Geometry check sheet. Reference: the model listing, model coordinates, mm. A direction names the side the tool comes from. Round coordinates to 2 decimals unless told otherwise and drop trailing zeros. Loops run counter-clockwise (first coordinate to the right, second up) from the corner with the lowest first, then second, coordinate; pieces in that order, holes last.
```python
from build123d import *

# Parameters (mm, degrees)
F1_DEPTH = 25.4
F2_DEPTH = 25.4
F3_DEPTH = 25.4


with BuildPart() as f1:
    # F0 (on Front) → F1 (new body)
    with BuildSketch(Plane.XZ):
        with BuildLine():
            ThreePointArc((-119.86399662, 0), (-111.5302178098, 16.6558061897), (-108.6615478184, 35.0579387173))
            ThreePointArc((-108.6615478184, 35.0579387173), (-111.4781642304, 53.2963683876), (-119.6655722325, 69.8354129505))
            Line((-119.6655722325, 69.8354129505), (-201.6532506958, 69.8354129505))
            Line((-201.6532506958, 69.8354129505), (-201.6532506958, 0))
            Line((-201.6532506958, 0), (-119.86399662, 0))
        make_face()
        with BuildLine():
            ThreePointArc((-119.6655722325, 69.8354129505), (-111.4781642304, 53.2963683876), (-108.6615478184, 35.0579387173))
            ThreePointArc((-108.6615478184, 35.0579387173), (-111.5302178098, 16.6558061897), (-119.86399662, 0))
            Line((-119.86399662, 0), (86.1022950306, 0))
            Line((86.1022950306, 0), (86.1022950306, 69.8354129505))
            Line((86.1022950306, 69.8354129505), (-119.6655722325, 69.8354129505))
        make_face()
        with BuildLine():
            Line((-201.6532506958, 69.8354129505), (-119.6655722325, 69.8354129505))
            ThreePointArc((-119.6655722325, 69.8354129505), (-229.5771812139, 35.2297180557), (-119.86399662, 0))
            Line((-119.86399662, 0), (-201.6532506958, 0))
            Line((-201.6532506958, 0), (-201.6532506958, 69.8354129505))
        make_face()
    extrude(amount=F1_DEPTH)

    # F2 (add): a face of the model
    f2_faces = [f1.faces().sort_by_distance(p)[0] for p in [
        (-83.8129637721, 0, 34.9783538695),
    ]]
    extrude(f2_faces, amount=F2_DEPTH)

    # F3 (cut): a face of the model
    f3_faces = [f1.faces().sort_by_distance(p)[0] for p in [
        (-83.8129637721, -25.4, 34.9783538695),
    ]]
    extrude(f3_faces, amount=-F3_DEPTH, mode=Mode.SUBTRACT)


solid = f1.part
```
1) Gauge pin test, flat ends, axial feed: pin 1 (1.5 mm diameter, centred on y = 6.5, z = 54, fed in from -X); pin 2 (2 mm diameter, centred on x = -57.5, y = 14, fed in from +Z); pin 3 (4 mm diameter, centred on y = 3.5, z = 34, fed in from -X). Record the tip position at first contact, or that the pin passes through.
Report:
pin 1: stops at x = -226.78
pin 2: stops at z = 69.84
pin 3: stops at x = -229.58
2) Access from +Z, -Z, +X, -X, +Y, -Y to the whole of each face (thin tool, end or side, straight path). Record for faces 1 (the face through (-18, 13, 0)), 2 (the face through (-15, 13, 69.835)), 3 (the face through (-74, 0, 36)).
Report:
face 1: -Z, +X, +Y, -Y
face 2: +Z, +X, +Y, -Y
face 3: +Z, -Z, +X, -X, -Y
3) Sectioned sample at B-B, the plane y = 9.75. Record the cut outline in (x, z).
Report:
outline: (-119.86, 0) - (86.1, 0) - (86.1, 69.84) - (-119.67, 69.84) arc R60.46 ccw (long way) to start
4) Scan lines: line 1 along Z through (x, y) = (-66.5, 4.5); line 2 along Z through (x, y) = (-167, 22.75); line 3 along X through (y, z) = (23.25, 48). Record each from-to range of solid material in increasing order.
Report:
line 1: z = 0 to 69.84
line 2: z = -25.36 to 95.48
line 3: x = -228.18 to 86.1
5) Sectioned sample at A-A, the plane x = -85. Record the cut outline in (y, z), then the cut area to 3 significant figures.
Report:
outline: (0, 0) - (25.4, 0) - (25.4, 69.84) - (0, 69.84) - close
area: 1,770 mm2
